The figure shows three views and two pictorial views of one solid part (mm, origin at its lowest corner). Answer the questions. A direction names the side the tool comes from. Give positions to 0.01 mm unless a question says otherwise; leave off trailing zeros. Order: outer loops, then holes, each group sorted by start corner. A loop starts at its lowest first (then second) coordinate and runs counter-clockwise, first axis right, second up. Notation, with made-up numbers: (1.5, 84) - (21.5, 84) arc R12 cw to (21.5, 106) - close; hole circle Ø1 at (87.25, 68). An arc over 180 degrees is marked (long way). Answer as a JSON object with one key per item and string values. Group by question number.
Q1. The mould has two halves that part along Y. Classify the marked faces 1, 2 and 3: released by +Y, released by -Y, zero draft, split by the parting line, or undercut.
Q2. Consider line 1 (Y direction, x = 15, z = 4.5); line 2 (X direction, y = 23, z = 1); line 3 (Y direction, x = 26, z = 6.5). Determine where each line is inside the solid, lowest interval first.
Q3. A cutting plane is placed at B-B, the plane x = 15. Give the vertices of the cut face in (y, z), and give its area (3 significant figures).
Q4. A cutting plane is placed at D-D, the plane x = 20. Give the vertices of the cut face in (y, z), and give its area (3 significant figures).
Q5. For the marked faces 4, 5 and 6, determine the directions among +Z, -Z, +X, -X, +Y, -Y from which every point of the face is accessible in a straight line to the end or side of a thin tool.
Q6. A cutting plane is placed at C-C, the plane z = 6.25. Give the vertices of the cut face in (x, y), and give its area (3 significant figures).
Q7. Given pin 1 (3 mm diameter, centred on y = 15.5, z = 1, fed in from -X); pin 2 (1.5 mm diameter, centred on y = 29.5, z = 3.5, fed in from +X); pin 3 (3.5 mm diameter, centred on x = 7.5, z = 2, fed in from +Y), each flat-ended and moving along its own axis, determine where each tip first touches the part or whether it passes through.
Q8. A cutting plane is placed at A-A, the plane y = 8. Give the vertices of the cut face in (x, z), and give its area (3 significant figures).
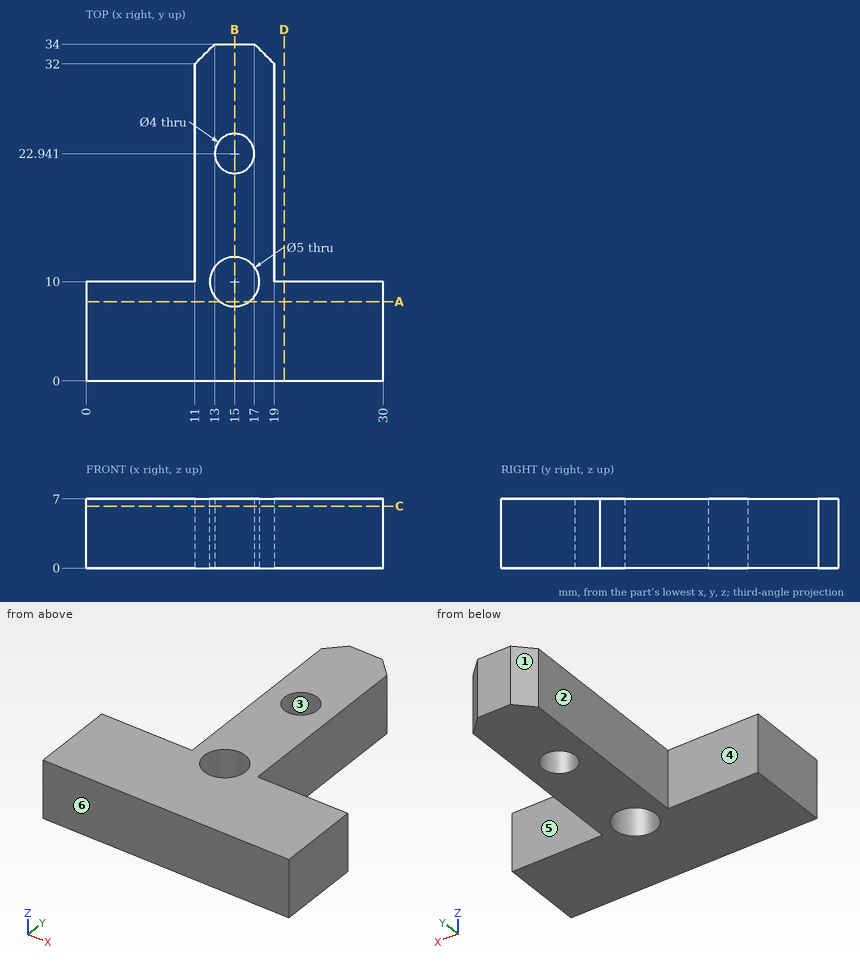
Reply:
{
 "1": {"face 1": "released by +Y", "face 2": "zero draft", "face 3": "undercut"},
 "2": {"line 1": "y = 0 to 7.5, 12.5 to 20.94, 24.94 to 34", "line 2": "x = 11 to 13, 17 to 19", "line 3": "y = 0 to 10"},
 "3": {"outline": "(0, 0) - (7.5, 0) - (7.5, 7) - (0, 7) - close; (12.5, 0) - (20.94, 0) - (20.94, 7) - (12.5, 7) - close; (24.94, 0) - (34, 0) - (34, 7) - (24.94, 7) - close", "area": "175 mm^2"},
 "4": {"outline": "(0, 0) - (10, 0) - (10, 7) - (0, 7) - close", "area": "70.0 mm^2"},
 "5": {"face 4": "+Z, -Z, -X, +Y", "face 5": "+Z, -Z, +X, +Y", "face 6": "+Z, -Z, +X, -X, -Y"},
 "6": {"outline": "(0, 0) - (30, 0) - (30, 10) - (19, 10) - (19, 32) - (17, 34) - (13, 34) - (11, 32) - (11, 10) - (0, 10) - close; hole circle Ø5 at (15, 10); hole circle Ø4 at (15, 22.94)", "area": "456 mm^2"},
 "7": {"pin 1": "stops at x = 11", "pin 2": "stops at x = 19", "pin 3": "stops at y = 10"},
 "8": {"outline": "(0, 0) - (13.5, 0) - (13.5, 7) - (0, 7) - close; (16.5, 0) - (30, 0) - (30, 7) - (16.5, 7) - close", "area": "189 mm^2"}
}
